Check sheet for the modelled part. Datum: model origin and axes. Units: mm. A direction names the side the tool comes from. Coordinates: 2 decimals unless noted, no trailing zeros. Loops run counter-clockwise (first coordinate to the right, second up) from the corner with the lowest first, then second, coordinate; pieces in that order, holes last. Notation, with made-up numbers: (-10, -27.75) - (29, -27.75) arc R18 ccw to (29, -1.75) - close; hole circle Ø3 at (80.25, 80.25). An arc over 180 degrees is marked (long way). Write each question's results on one line, items separated by ' | '. Start each with the question number.
1. Cross-section at D-D (z = 11). Record the cut outline in (x, y), and give its area (3 significant figures).
2. Tool access check on faces 1 (the face through (-11, 0, 4.5)), 2 (the face through (16, -1, 4.5)), 3 (the face through (-9.844, -0.575, 2.979)). Record the directions out of +Z, -Z, +X, -X, +Y, -Y that give a thin tool (end or side, any length) a straight path to the whole face; none if there is none.
3. Draft check along Y on faces 4 (the face through (15.09, -6.81, 2.98)), 5 (the face through (-3.933, 0, 9)), 6 (the face through (14.78, 4.17, 2.98)), 7 (the face through (2, 12.689, 1)). Enter one of: released by +Y, released by -Y, zero draft, split by the parting line, or undercut.
4. Cross-section at A-A (x = 16). Record the cut outline in (y, z).
5. Thickness scan on line 1 (Y direction, x = 13.5, z = 9.25); line 2 (X direction, y = -5, z = 5); line 3 (Z direction, x = 6.5, y = 9). Record the ranges inside material, lowest first. Write a range as [from, to].
6. Cross-section at B-B (y = 5). Record the cut outline in (x, z), and give its area (3 significant figures).
7. Cross-section at C-C (x = 8). Record the cut outline in (y, z).
8. Gauge pin test, flat ends, axial feed: P1, Ø6, axis at x = -8, y = 1.5, coming from the +Z side; P2, Ø4, axis at x = 16.53, y = 10.07, coming from the +Z side; P3, Ø4.5, axis at y = 3, z = 7.5, coming from the -X side; P4, Ø1.8, axis at x = -11.48, y = -10.43, coming from the +Z side. Record the tip position at first contact, or that the pin passes through.
```python
from build123d import *

# Parameters (mm, degrees)
SKETCH_1_W      = 33.51
SKETCH_1_H      = 25.73
SKETCH_1_R      = 1.5
EXTRUDE_1_DEPTH = 1.5
SKETCH_2_W      = 18
SKETCH_2_H      = 15
EXTRUDE_2_DEPTH = 15
SKETCH_3_R      = 1.5
EXTRUDE_3_DEPTH = 3


with BuildPart() as part:
    # 草圖1 → 填料-伸長1 (new body)
    with BuildSketch(Plane.XY):
        with Locations((2.525137649, -0.176232877)):
            Rectangle(SKETCH_1_W, SKETCH_1_H)
        with Locations((-11.474862351, 10.073766514)):
            Circle(SKETCH_1_R, mode=Mode.SUBTRACT)
        with Locations((-11.479862351, -10.426232877)):
            Circle(SKETCH_1_R, mode=Mode.SUBTRACT)
        with Locations((16.520137649, -10.426232877)):
            Circle(SKETCH_1_R, mode=Mode.SUBTRACT)
        with Locations((16.525137649, 10.073766514)):
            Circle(SKETCH_1_R, mode=Mode.SUBTRACT)
    extrude(amount=EXTRUDE_1_DEPTH)

    # 草圖2 → 填料-伸長2 (add)
    with BuildSketch(Plane.XY.offset(1.5)):
        with Locations((5.066714054, -0.011232877)):
            Rectangle(SKETCH_2_W, SKETCH_2_H)
    extrude(amount=EXTRUDE_2_DEPTH)

    # 草圖3 → 填料-伸長3 (add)
    with BuildSketch(Plane.XY.offset(1.5)):
        with Locations((-11.229862351, 5)):
            Circle(SKETCH_3_R)
        with Locations((-11.229862351, 0)):
            Circle(SKETCH_3_R)
        with Locations((-11.229862351, -5)):
            Circle(SKETCH_3_R)
        with Locations((16.280137649, 4.100671386)):
            Circle(SKETCH_3_R)
        with Locations((16.280137649, -0.899328614)):
            Circle(SKETCH_3_R)
        with Locations((16.280137649, -5.899328614)):
            Circle(SKETCH_3_R)
    extrude(amount=EXTRUDE_3_DEPTH)


solid = part.part
```
Established:
1) outline: (-3.93, -7.51) - (14.07, -7.51) - (14.07, 7.49) - (-3.93, 7.49) - close | area: 270 mm^2
2) face 1: +Z, -X, +Y, -Y | face 2: +Z, +X, +Y, -Y | face 3: +Z
3) face 4: undercut | face 5: zero draft | face 6: undercut | face 7: released by +Y
4) outline: (-13.04, 0) - (-11.83, 0) - (-11.83, 1.5) - (-13.04, 1.5) - close; (-9.02, 0) - (8.67, 0) - (8.67, 1.5) - (5.57, 1.5) - (5.57, 4.5) - (2.63, 4.5) - (2.63, 1.5) - (0.57, 1.5) - (0.57, 4.5) - (-2.37, 4.5) - (-2.37, 1.5) - (-4.43, 1.5) - (-4.43, 4.5) - (-7.37, 4.5) - (-7.37, 1.5) - (-9.02, 1.5) - close; (11.48, 0) - (12.69, 0) - (12.69, 1.5) - (11.48, 1.5) - close
5) line 1: [-7.51, 7.49] | line 2: [-3.93, 14.07] | line 3: [0, 1.5]
6) outline: (-14.23, 0) - (19.28, 0) - (19.28, 1.5) - (17.48, 1.5) - (17.48, 4.5) - (15.08, 4.5) - (15.08, 1.5) - (14.07, 1.5) - (14.07, 16.5) - (-3.93, 16.5) - (-3.93, 1.5) - (-9.73, 1.5) - (-9.73, 4.5) - (-12.73, 4.5) - (-12.73, 1.5) - (-14.23, 1.5) - close | area: 336 mm^2
7) outline: (-13.04, 0) - (12.69, 0) - (12.69, 1.5) - (7.49, 1.5) - (7.49, 16.5) - (-7.51, 16.5) - (-7.51, 1.5) - (-13.04, 1.5) - close
8) P1: z = 4.5 | P2: z = 1.5 | P3: x = -3.93 | P4: through
